from build123d import *

# Parameters (mm, degrees)
EXTRUDE_1_DEPTH               = 3
HOLE_WIZARD_M2_1_AT_2_COUNT   = 2
HOLE_WIZARD_M2_1_AT_2_PITCH   = 21
PATTERN_LINEAR_1_COUNT        = 3
PATTERN_LINEAR_1_PITCH        = 33
PATTERN_LINEAR_2_COUNT        = 3
PATTERN_LINEAR_2_PITCH        = 10.5
PATTERN_LINEAR_3_COUNT        = 2
PATTERN_LINEAR_3_PITCH        = 31.5
HOLE_WIZARD_M2_1_2_AT_2_COUNT = 2
HOLE_WIZARD_M2_1_2_AT_2_PITCH = 16.970562748
SKETCH_8_R                    = 17
CUT_EXTRUDE_1_DEPTH           = 1
SKETCH_9_R                    = 2.025
CUT_EXTRUDE_2_DEPTH           = 75.994999833
PATTERN_CIRCULAR_1_COUNT      = 2
PATTERN_CIRCULAR_1_ANGLE      = 90
FILLET_1_R                    = 4
CUT_EXTRUDE_3_DEPTH           = 76.028327984
CHAMFER_2_SIZE                = 1


with BuildPart() as part:
    # ｽｹｯﾁ1 → ﾎﾞｽ - 押し出し1 (new body)
    with BuildSketch(Plane(origin=(0, 0, 0), x_dir=(1, 0, 0), z_dir=(0, 1, 0))):
        with BuildLine():
            Line((-10.05, 0), (-39, 0))
            Line((-39, 0), (-47.5, 8.5))
            Line((-47.5, 8.5), (-47.5, 58))
            Line((-47.5, 58), (47.5, 58))
            Line((47.5, 58), (47.5, 8.5))
            Line((47.5, 8.5), (39, 0))
            Line((39, 0), (10.05, 0))
            ThreePointArc((10.05, 0), (0, 10.05), (-10.05, 0))
        make_face()
    extrude(amount=EXTRUDE_1_DEPTH)

    # ｽｹｯﾁ3 → Hole Wizard M2 _1 (revolve, cut)
    with BuildSketch(Plane(origin=(-43.5, 3, -54), x_dir=(0, 0, 1), z_dir=(1, 0, 0))):
        Polygon((0, 0), (0, 4.63090365), (1.05, 4), (1.05, 1), (2, 1), (2, 0), align=None)
    hole_wizard_m2_1 = revolve(axis=Axis((-43.5, 9.35, -54), (0, -1, 0)), mode=Mode.SUBTRACT)

    # Hole Wizard M2 _1 at 2: Hole Wizard M2 _1 ×2
    with Locations(*[(i * HOLE_WIZARD_M2_1_AT_2_PITCH, 0, 0) for i in range(1, HOLE_WIZARD_M2_1_AT_2_COUNT)]):
        add(hole_wizard_m2_1, mode=Mode.SUBTRACT)

    # 直線ﾊﾟﾀｰﾝ1: Hole Wizard M2 _1 ×3
    with Locations(*[(i * PATTERN_LINEAR_1_PITCH, 0, 0) for i in range(1, PATTERN_LINEAR_1_COUNT)]):
        add(hole_wizard_m2_1, mode=Mode.SUBTRACT)

    # 直線ﾊﾟﾀｰﾝ1 copy 1 sketch → 直線ﾊﾟﾀｰﾝ1 copy 1 (revolve, cut)
    with BuildSketch(Plane(origin=(10.5, 3, -54), x_dir=(0, 0, 1), z_dir=(1, 0, 0))):
        Polygon((0, 0), (0, 4.63090365), (1.05, 4), (1.05, 1), (2, 1), (2, 0), align=None)
    revolve(axis=Axis((10.5, 9.35, -54), (0, -1, 0)), mode=Mode.SUBTRACT)

    # 直線ﾊﾟﾀｰﾝ1 copy 2 sketch → 直線ﾊﾟﾀｰﾝ1 copy 2 (revolve, cut)
    with BuildSketch(Plane(origin=(43.5, 3, -54), x_dir=(0, 0, 1), z_dir=(1, 0, 0))):
        Polygon((0, 0), (0, 4.63090365), (1.05, 4), (1.05, 1), (2, 1), (2, 0), align=None)
    revolve(axis=Axis((43.5, 9.35, -54), (0, -1, 0)), mode=Mode.SUBTRACT)

    # 直線ﾊﾟﾀｰﾝ2: Hole Wizard M2 _1 ×3
    with Locations(*[(0, 0, i * PATTERN_LINEAR_2_PITCH) for i in range(1, PATTERN_LINEAR_2_COUNT)]):
        add(hole_wizard_m2_1, mode=Mode.SUBTRACT)

    # 直線ﾊﾟﾀｰﾝ2 copy 1 sketch → 直線ﾊﾟﾀｰﾝ2 copy 1 (revolve, cut)
    with BuildSketch(Plane(origin=(-22.5, 3, -43.5), x_dir=(0, 0, 1), z_dir=(1, 0, 0))):
        Polygon((0, 0), (0, 4.63090365), (1.05, 4), (1.05, 1), (2, 1), (2, 0), align=None)
    revolve(axis=Axis((-22.5, 9.35, -43.5), (0, -1, 0)), mode=Mode.SUBTRACT)

    # 直線ﾊﾟﾀｰﾝ2 copy 2 sketch → 直線ﾊﾟﾀｰﾝ2 copy 2 (revolve, cut)
    with BuildSketch(Plane(origin=(-22.5, 3, -33), x_dir=(0, 0, 1), z_dir=(1, 0, 0))):
        Polygon((0, 0), (0, 4.63090365), (1.05, 4), (1.05, 1), (2, 1), (2, 0), align=None)
    revolve(axis=Axis((-22.5, 9.35, -33), (0, -1, 0)), mode=Mode.SUBTRACT)

    # 直線ﾊﾟﾀｰﾝ2 copy 3 sketch → 直線ﾊﾟﾀｰﾝ2 copy 3 (revolve, cut)
    with BuildSketch(Plane(origin=(-10.5, 3, -43.5), x_dir=(0, 0, 1), z_dir=(1, 0, 0))):
        Polygon((0, 0), (0, 4.63090365), (1.05, 4), (1.05, 1), (2, 1), (2, 0), align=None)
    revolve(axis=Axis((-10.5, 9.35, -43.5), (0, -1, 0)), mode=Mode.SUBTRACT)

    # 直線ﾊﾟﾀｰﾝ2 copy 4 sketch → 直線ﾊﾟﾀｰﾝ2 copy 4 (revolve, cut)
    with BuildSketch(Plane(origin=(-10.5, 3, -33), x_dir=(0, 0, 1), z_dir=(1, 0, 0))):
        Polygon((0, 0), (0, 4.63090365), (1.05, 4), (1.05, 1), (2, 1), (2, 0), align=None)
    revolve(axis=Axis((-10.5, 9.35, -33), (0, -1, 0)), mode=Mode.SUBTRACT)

    # 直線ﾊﾟﾀｰﾝ2 copy 5 sketch → 直線ﾊﾟﾀｰﾝ2 copy 5 (revolve, cut)
    with BuildSketch(Plane(origin=(22.5, 3, -43.5), x_dir=(0, 0, 1), z_dir=(1, 0, 0))):
        Polygon((0, 0), (0, 4.63090365), (1.05, 4), (1.05, 1), (2, 1), (2, 0), align=None)
    revolve(axis=Axis((22.5, 9.35, -43.5), (0, -1, 0)), mode=Mode.SUBTRACT)

    # 直線ﾊﾟﾀｰﾝ2 copy 6 sketch → 直線ﾊﾟﾀｰﾝ2 copy 6 (revolve, cut)
    with BuildSketch(Plane(origin=(22.5, 3, -33), x_dir=(0, 0, 1), z_dir=(1, 0, 0))):
        Polygon((0, 0), (0, 4.63090365), (1.05, 4), (1.05, 1), (2, 1), (2, 0), align=None)
    revolve(axis=Axis((22.5, 9.35, -33), (0, -1, 0)), mode=Mode.SUBTRACT)

    # 直線ﾊﾟﾀｰﾝ2 copy 7 sketch → 直線ﾊﾟﾀｰﾝ2 copy 7 (revolve, cut)
    with BuildSketch(Plane(origin=(10.5, 3, -43.5), x_dir=(0, 0, 1), z_dir=(1, 0, 0))):
        Polygon((0, 0), (0, 4.63090365), (1.05, 4), (1.05, 1), (2, 1), (2, 0), align=None)
    revolve(axis=Axis((10.5, 9.35, -43.5), (0, -1, 0)), mode=Mode.SUBTRACT)

    # 直線ﾊﾟﾀｰﾝ2 copy 8 sketch → 直線ﾊﾟﾀｰﾝ2 copy 8 (revolve, cut)
    with BuildSketch(Plane(origin=(10.5, 3, -33), x_dir=(0, 0, 1), z_dir=(1, 0, 0))):
        Polygon((0, 0), (0, 4.63090365), (1.05, 4), (1.05, 1), (2, 1), (2, 0), align=None)
    revolve(axis=Axis((10.5, 9.35, -33), (0, -1, 0)), mode=Mode.SUBTRACT)

    # 直線ﾊﾟﾀｰﾝ2 copy 9 sketch → 直線ﾊﾟﾀｰﾝ2 copy 9 (revolve, cut)
    with BuildSketch(Plane(origin=(43.5, 3, -43.5), x_dir=(0, 0, 1), z_dir=(1, 0, 0))):
        Polygon((0, 0), (0, 4.63090365), (1.05, 4), (1.05, 1), (2, 1), (2, 0), align=None)
    revolve(axis=Axis((43.5, 9.35, -43.5), (0, -1, 0)), mode=Mode.SUBTRACT)

    # 直線ﾊﾟﾀｰﾝ2 copy 10 sketch → 直線ﾊﾟﾀｰﾝ2 copy 10 (revolve, cut)
    with BuildSketch(Plane(origin=(43.5, 3, -33), x_dir=(0, 0, 1), z_dir=(1, 0, 0))):
        Polygon((0, 0), (0, 4.63090365), (1.05, 4), (1.05, 1), (2, 1), (2, 0), align=None)
    revolve(axis=Axis((43.5, 9.35, -33), (0, -1, 0)), mode=Mode.SUBTRACT)

    # 直線ﾊﾟﾀｰﾝ3: Hole Wizard M2 _1 ×2
    with Locations(*[(0, 0, i * PATTERN_LINEAR_3_PITCH) for i in range(1, PATTERN_LINEAR_3_COUNT)]):
        add(hole_wizard_m2_1, mode=Mode.SUBTRACT)

    # 直線ﾊﾟﾀｰﾝ3 copy 1 sketch → 直線ﾊﾟﾀｰﾝ3 copy 1 (revolve, cut)
    with BuildSketch(Plane(origin=(-22.5, 3, -22.5), x_dir=(0, 0, 1), z_dir=(1, 0, 0))):
        Polygon((0, 0), (0, 4.63090365), (1.05, 4), (1.05, 1), (2, 1), (2, 0), align=None)
    revolve(axis=Axis((-22.5, 9.35, -22.5), (0, -1, 0)), mode=Mode.SUBTRACT)

    # ｽｹｯﾁ5 → Hole Wizard M2 _1 2 (revolve, cut)
    with BuildSketch(Plane(origin=(-10.5, 3, -22.5), x_dir=(0, 0, 1), z_dir=(1, 0, 0))):
        Polygon((0, 0), (0, 6.480688495), (0.8, 6), (0.8, 0), align=None)
    hole_wizard_m2_1_2 = revolve(axis=Axis((-10.5, 9.35, -22.5), (0, -1, 0)), mode=Mode.SUBTRACT)

    # Hole Wizard M2 _1 2 at 2: Hole Wizard M2 _1 2 ×2
    with Locations(*[Vector(-0.7071067811865469, 0, 0.7071067811865482) * (i * HOLE_WIZARD_M2_1_2_AT_2_PITCH) for i in range(1, HOLE_WIZARD_M2_1_2_AT_2_COUNT)]):
        add(hole_wizard_m2_1_2, mode=Mode.SUBTRACT)

    # ｽｹｯﾁ7 → M2 なべ頭ねじ用座ぐり穴2 (revolve, cut)
    with BuildSketch(Plane(origin=(-43.5, 3, -12), x_dir=(0, 0, 1), z_dir=(1, 0, 0))):
        Polygon((0, 0), (0, 6.63090365), (1.05, 6), (1.05, 1), (2, 1), (2, 0), align=None)
    hole_wizard_m2_2 = revolve(axis=Axis((-43.5, 9.35, -12), (0, -1, 0)), mode=Mode.SUBTRACT)

    # ﾐﾗｰ1: Hole Wizard M2 _1 2, M2 なべ頭ねじ用座ぐり穴2 across plane
    add(hole_wizard_m2_1_2.mirror(Plane(origin=(0, 0, 0), x_dir=(0, 0, 1), z_dir=(1, 0, 0))), mode=Mode.SUBTRACT)
    add(hole_wizard_m2_2.mirror(Plane(origin=(0, 0, 0), x_dir=(0, 0, 1), z_dir=(1, 0, 0))), mode=Mode.SUBTRACT)

    # ﾐﾗｰ1 copy 1 sketch → ﾐﾗｰ1 copy 1 (revolve, cut)
    with BuildSketch(Plane(origin=(43.5, 3, -22.5), x_dir=(0, 0, 1), z_dir=(-1, 0, 0))):
        Polygon((0, 0), (0, -4.63090365), (1.05, -4), (1.05, -1), (2, -1), (2, 0), align=None)
    revolve(axis=Axis((43.5, 9.35, -22.5), (0, 1, 0)), mode=Mode.SUBTRACT)

    # ﾐﾗｰ1 copy 2 sketch → ﾐﾗｰ1 copy 2 (revolve, cut)
    with BuildSketch(Plane(origin=(22.5, 3, -22.5), x_dir=(0, 0, 1), z_dir=(-1, 0, 0))):
        Polygon((0, 0), (0, -4.63090365), (1.05, -4), (1.05, -1), (2, -1), (2, 0), align=None)
    revolve(axis=Axis((22.5, 9.35, -22.5), (0, 1, 0)), mode=Mode.SUBTRACT)

    # ﾐﾗｰ1 copy 3 sketch → ﾐﾗｰ1 copy 3 (revolve, cut)
    with BuildSketch(Plane(origin=(43.5, 3, -54), x_dir=(0, 0, 1), z_dir=(-1, 0, 0))):
        Polygon((0, 0), (0, -4.63090365), (1.05, -4), (1.05, -1), (2, -1), (2, 0), align=None)
    revolve(axis=Axis((43.5, 9.35, -54), (0, 1, 0)), mode=Mode.SUBTRACT)

    # ﾐﾗｰ1 copy 4 sketch → ﾐﾗｰ1 copy 4 (revolve, cut)
    with BuildSketch(Plane(origin=(22.5, 3, -54), x_dir=(0, 0, 1), z_dir=(-1, 0, 0))):
        Polygon((0, 0), (0, -4.63090365), (1.05, -4), (1.05, -1), (2, -1), (2, 0), align=None)
    revolve(axis=Axis((22.5, 9.35, -54), (0, 1, 0)), mode=Mode.SUBTRACT)

    # ﾐﾗｰ1 copy 5 sketch → ﾐﾗｰ1 copy 5 (revolve, cut)
    with BuildSketch(Plane(origin=(22.5, 3, -10.5), x_dir=(0, 0, 1), z_dir=(-1, 0, 0))):
        Polygon((0, 0), (0, -6.480688495), (0.8, -6), (0.8, 0), align=None)
    revolve(axis=Axis((22.5, 9.35, -10.5), (0, 1, 0)), mode=Mode.SUBTRACT)

    # ｽｹｯﾁ8 → ｶｯﾄ - 押し出し1 (cut)
    with BuildSketch(Plane(origin=(0, 3, 0), x_dir=(1, 0, 0), z_dir=(0, 1, 0))):
        Circle(SKETCH_8_R)
    extrude(amount=-CUT_EXTRUDE_1_DEPTH, mode=Mode.SUBTRACT)

    # ｽｹｯﾁ9 → ｶｯﾄ - 押し出し2 (cut, through all)
    with BuildSketch(Plane(origin=(0, 2, 0), x_dir=(1, 0, 0), z_dir=(0, 1, 0))):
        with Locations(Location((-9.899494937, 9.899494937, 0), (0, 0, 270))):
            Circle(SKETCH_9_R)
    cut_extrude_2 = extrude(amount=-CUT_EXTRUDE_2_DEPTH, mode=Mode.SUBTRACT)

    # 円形ﾊﾟﾀｰﾝ1: ｶｯﾄ - 押し出し2 ×2 about axis
    pattern_circular_1_axis = Axis((0, 3, 0), (0, -1, 0))
    for i in range(1, PATTERN_CIRCULAR_1_COUNT):
        add(cut_extrude_2.rotate(pattern_circular_1_axis, i * PATTERN_CIRCULAR_1_ANGLE / (PATTERN_CIRCULAR_1_COUNT - 1)), mode=Mode.SUBTRACT)

    # ﾌｨﾚｯﾄ1
    fillet_1_edges = [part.edges().sort_by_distance(p)[0] for p in [
        (-47.5, 1.5, -8.5),
        (-47.5, 1.5, -58),
        (47.5, 1.5, -58),
        (47.5, 1.5, -8.5),
        (39, 1.5, 0),
        (-39, 1.5, 0),
    ]]
    fillet(fillet_1_edges, radius=FILLET_1_R)

    # ｽｹｯﾁ10 → ｶｯﾄ - 押し出し3 (cut, through all)
    with BuildSketch(Plane(origin=(0, 3, 0), x_dir=(1, 0, 0), z_dir=(0, 1, 0))):
        with BuildLine():
            Line((-47.5, 0), (-21, 0))
            ThreePointArc((-21, 0), (0, 21), (21, 0))
            Line((21, 0), (47.5, 0))
            Line((47.5, 0), (47.5, 58))
            Line((47.5, 58), (-47.5, 58))
            Line((-47.5, 58), (-47.5, 0))
        make_face()
    extrude(amount=-CUT_EXTRUDE_3_DEPTH, mode=Mode.SUBTRACT)

    # 面取り2
    chamfer_2_edges = [part.edges().sort_by_distance(p)[0] for p in [
        (19, 3, 0),
        (0, 3, -17),
        (-19, 3, 0),
        (0, 3, -21),
    ]]
    chamfer(chamfer_2_edges, length=CHAMFER_2_SIZE - 0.0001)  # a hair under: the kernel refuses the full size


solid = part.part
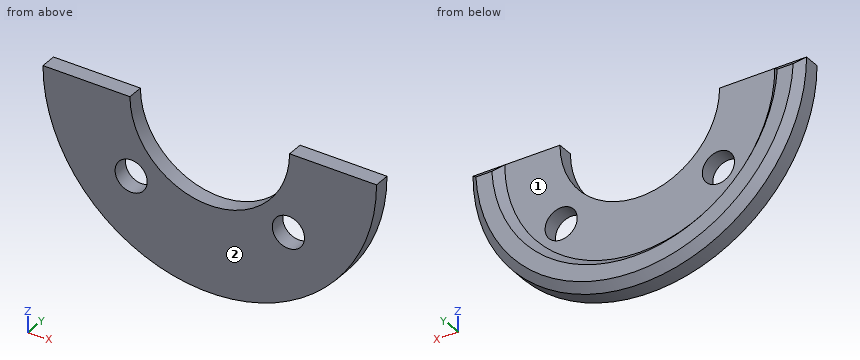
Work out the finished part from the listing and answer in its coordinate system (mm). Face numbers are marked on the shaded views. Round coordinates to 2 decimals unless told otherwise and drop trailing zeros. One line per item, written item: value.
Q1. Straight lines are drawn through the part: line 1 (X direction, y = 1.3, z = -8.75); line 2 (Y direction, x = 10.5, z = -3.75); line 3 (X direction, y = 2.8, z = -12). For each, find the intervals that lie inside material, in ascending order.
Derived:
line 1: -19.09 to -11.57, -8.23 to -4.94, 4.94 to 8.23, 11.57 to 19.09
line 2: 0 to 2
line 3: -16.25 to -13.15, 13.15 to 16.25
Q2. Find section B-B on y = 1.25. Give the number of separate pieces and of enclosed holes in the cut face, then the cut area to 3 significant figures.
Derived:
separate pieces: 1
enclosed holes: 2
area: 508 mm²
Q3. A flat-ended cylindrical pin translates along its axis: pin 1 (1.5 mm diameter, centred on x = -1, z = -14, fed in from +Y). Find the tip coordinate at first contact, or state that the pin passes through.
Derived:
pin 1: y = 2
Q4. Determine the mould class of the marked faces 1 and 2 for opening direction X: released by +X, released by -X, zero draft, split by the parting line, or undercut.
Derived:
face 1: undercut
face 2: zero draft
